Design review of the part built by this model. Coordinates are the model's own, in mm. A direction names the side the tool comes from. Coordinates: 2 decimals unless noted, no trailing zeros. Write each loop counter-clockwise with the first axis right and the second up, starting at its lowest first coordinate (ties: lowest second). Pieces come first, ordered by that corner, then holes.
Q1. Take a section at C-C (z = 6). Give the boundary of the cut face in (x, y).
Q2. Machinability: for faces 4 (the flat face through (-48.5, 6, -7)), 5 (the flat face through (3, 2, 5)), which of the approach directions +Z, -Z, +X, -X, +Y, -Y give a long, thin tool a straight path to every point of the face, cutting with its end or side? Answer none if there is none.
Q3. Take a section at B-B (x = -54.5). Give the boundary of the cut face in (y, z), and give its area (3 significant figures).
Q4. For probe 1 along Y at (x, z) = (-54.5, 7.45); probe 2 along Y at (x, z) = (-4, 0.75); probe 3 along Z at (x, y) = (-53, 6.75), list the stretches that pass through material, from the lowest coordinate up.
Q5. Take a section at A-A (y = 7). Give the boundary of the cut face in (x, z), and give its area (3 significant figures).
Q6. Mouldability with a two-part tool opening along X and no side actions: class faces 1 (the flat face through (-48.5, 6, 7)), 2 (the flat face through (-52, 4, -5)), 3 (the cylindrical face through (-53, 4, 7)) as pulls with the +X half, pulls with the -X half, needs draft (parallel to the pull), parting line crosses it, or undercut.
Q7. Insertion check: pin 1 (2 mm diameter, centred on x = 26.5, y = 2, fed in from -Z); pin 2 (4 mm diameter, centred on x = -5, y = 3, fed in from +Z); pin 3 (8 mm diameter, centred on x = 22.5, z = 0, fed in from +Y). Each pin has a flat end and moves straight along its axis. Give the tip position at first contact, or say it passes through.
```python
from build123d import *

# Parameters (mm, degrees)
SZKIC1_W                         = 101
SZKIC1_H                         = 10
DODANIE_WYCI_GNI_CIE1_DEPTH      = 4
DODANIE_WYCI_GNI_CIE2_DEPTH      = 8
DODANIE_WYCI_GNI_CIE2_DEPTH_BACK = 4
SZKIC2_W                         = 4
SZKIC2_H                         = 8
SFAZOWANIE1_SIZE                 = 4
SFAZOWANIE2_SIZE                 = 4
WYTNIJ_WYCI_GNI_CIE1_DEPTH       = 62.72722252
WYTNIJ_WYCI_GNI_CIE1_DEPTH_BACK  = 62.72722252
SZKIC4_R                         = 1.5
SFAZOWANIE3_SIZE                 = 2


# Some blends are built 0.0001 mm under size
with BuildPart() as part:
    # Szkic1 → Dodanie-wyciągnięcie1 (new body)
    with BuildSketch(Plane(origin=(0, 0, 0), x_dir=(1, 0, 0), z_dir=(0, 1, 0))):
        Rectangle(SZKIC1_W, SZKIC1_H)
    extrude(amount=DODANIE_WYCI_GNI_CIE1_DEPTH)

    # Szkic2 → Dodanie-wyciągnięcie2 (add, two sides: drawn at the far end of the back side and taken through both)
    with BuildSketch(Plane.ZY.offset(50.5).offset(-DODANIE_WYCI_GNI_CIE2_DEPTH_BACK)):
        with Locations((-7, 4)):
            Rectangle(SZKIC2_W, SZKIC2_H)
        with Locations((7, 4)):
            Rectangle(SZKIC2_W, SZKIC2_H)
    extrude(amount=DODANIE_WYCI_GNI_CIE2_DEPTH + DODANIE_WYCI_GNI_CIE2_DEPTH_BACK)

    # Sfazowanie1
    sfazowanie1_edges = [part.edges().sort_by_distance(p)[0] for p in [
        (-46.5, 8, -7),
        (-46.5, 8, 7),
    ]]
    chamfer(sfazowanie1_edges, length=SFAZOWANIE1_SIZE)

    # Sfazowanie2
    # the kernel refuses this chamfer: 4 mm, written as the material it adds along each edge
    with BuildSketch(Plane(origin=(-46.5, 0, -5), x_dir=(0.9996219169112968, 0, 0.027495876610586296), z_dir=(0, 1, 0))) as sfazowanie2_piece_1_section:
        Polygon((SFAZOWANIE2_SIZE * 0.999621916911, SFAZOWANIE2_SIZE * 0.0274958766106), (-SFAZOWANIE2_SIZE * 0.0274958766106, SFAZOWANIE2_SIZE * 0.999621916911), (0, 0), align=None)
    sfazowanie2_piece_1 = extrude(amount=4, mode=Mode.PRIVATE)
    sfazowanie2_piece_1 = split(sfazowanie2_piece_1, bisect_by=Plane(origin=(-45.556052557, 1.526245094, -9), z_dir=(0, 0, 1)), keep=Keep.TOP, mode=Mode.PRIVATE)
    sfazowanie2_piece_1 = split(sfazowanie2_piece_1, bisect_by=Plane(origin=(-44.791148825, 2.291148825, -6.514062333), z_dir=(-0.7071067811865476, -0.7071067811865476, 0)), keep=Keep.TOP, mode=Mode.PRIVATE)
    add(sfazowanie2_piece_1)
    with BuildSketch(Plane(origin=(-46.5, 0, -5), x_dir=(0.9996219169112968, 0, 0.027495876610586296), z_dir=(0, 1, 0))) as sfazowanie2_piece_2_section:
        Polygon((SFAZOWANIE2_SIZE * 0.999621916911, SFAZOWANIE2_SIZE * 0.0274958766106), (-SFAZOWANIE2_SIZE * 0.0274958766106, SFAZOWANIE2_SIZE * 0.999621916911), (0, 0), align=None)
    sfazowanie2_piece_2 = extrude(amount=4, mode=Mode.PRIVATE)
    sfazowanie2_piece_2 = split(sfazowanie2_piece_2, bisect_by=Plane(origin=(-44.936302596, 2.436302596, -5.911229734), z_dir=(0.7071067811865476, 0.7071067811865476, 0)), keep=Keep.TOP, mode=Mode.PRIVATE)
    add(sfazowanie2_piece_2)
    with BuildSketch(Plane(origin=(-46.5, 4, 5), x_dir=(-0.027495876610585623, 0, 0.9996219169112968), z_dir=(0, -1, 0))) as sfazowanie2_piece_3_section:
        Polygon((SFAZOWANIE2_SIZE * 0.999621916911, -SFAZOWANIE2_SIZE * 0.0274958766106), (-SFAZOWANIE2_SIZE * 0.0274958766106, -SFAZOWANIE2_SIZE * 0.999621916911), (0, 0), align=None)
    sfazowanie2_piece_3 = extrude(amount=4, mode=Mode.PRIVATE)
    sfazowanie2_piece_3 = split(sfazowanie2_piece_3, bisect_by=Plane(origin=(-44.936302596, 2.436302596, 5.911229734), z_dir=(0.7071067811865476, 0.7071067811865476, 0)), keep=Keep.TOP, mode=Mode.PRIVATE)
    add(sfazowanie2_piece_3)
    with BuildSketch(Plane(origin=(-46.5, 4, 5), x_dir=(-0.027495876610585623, 0, 0.9996219169112968), z_dir=(0, -1, 0))) as sfazowanie2_piece_4_section:
        Polygon((SFAZOWANIE2_SIZE * 0.999621916911, -SFAZOWANIE2_SIZE * 0.0274958766106), (-SFAZOWANIE2_SIZE * 0.0274958766106, -SFAZOWANIE2_SIZE * 0.999621916911), (0, 0), align=None)
    sfazowanie2_piece_4 = extrude(amount=4, mode=Mode.PRIVATE)
    sfazowanie2_piece_4 = split(sfazowanie2_piece_4, bisect_by=Plane(origin=(-45.556052557, 1.526245094, 9), z_dir=(0, 0, -1)), keep=Keep.TOP, mode=Mode.PRIVATE)
    sfazowanie2_piece_4 = split(sfazowanie2_piece_4, bisect_by=Plane(origin=(-44.791148825, 2.291148825, 6.514062333), z_dir=(-0.7071067811865476, -0.7071067811865476, 0)), keep=Keep.TOP, mode=Mode.PRIVATE)
    add(sfazowanie2_piece_4)

    # Szkic4 → Wytnij-wyciągnięcie1 (cut, two sides: drawn at the far end of the back side and taken through both)
    with BuildSketch(Plane.XY.offset(9).offset(-WYTNIJ_WYCI_GNI_CIE1_DEPTH_BACK)):
        with Locations((-54.5, 4)):
            Circle(SZKIC4_R)
    extrude(amount=WYTNIJ_WYCI_GNI_CIE1_DEPTH + WYTNIJ_WYCI_GNI_CIE1_DEPTH_BACK, mode=Mode.SUBTRACT)

    # Sfazowanie3
    sfazowanie3_edges = [part.edges().sort_by_distance(p)[0] for p in [
        (50.5, 4, 0),
        (50.5, 0, 0),
    ]]
    chamfer(sfazowanie3_edges, length=SFAZOWANIE3_SIZE - 0.0001)  # a hair under: the kernel refuses the full size


solid = part.part
```
Response:
1. outline: (-58.5, 0) - (-43.5, 0) - (-43.5, 4) - (-46.5, 4) - (-50.5, 8) - (-58.5, 8) - close; hole circle Ø3 at (-54.5, 4)
2. face 4: +Z, -Z, +X, +Y
2. face 5: +Z, +X, +Y, -Y
3. outline: (0, -9) - (2.5, -9) - (2.5, -5) - (0, -5) - close; (0, 5) - (2.5, 5) - (2.5, 9) - (0, 9) - close; (5.5, -9) - (8, -9) - (8, -5) - (5.5, -5) - close; (5.5, 5) - (8, 5) - (8, 9) - (5.5, 9) - close
3. area: 40.0 mm2
4. probe 1: y = 0 to 2.5, 5.5 to 8
4. probe 2: y = 0 to 4
4. probe 3: z = -9 to -5, 5 to 9
5. outline: (-58.5, -9) - (-49.5, -9) - (-49.5, -5) - (-58.5, -5) - close; (-58.5, 5) - (-49.5, 5) - (-49.5, 9) - (-58.5, 9) - close
5. area: 72.0 mm2
6. face 1: pulls with the +X half
6. face 2: needs draft
6. face 3: undercut
7. pin 1: stops at z = -5
7. pin 2: stops at z = 5
7. pin 3: stops at y = 4
